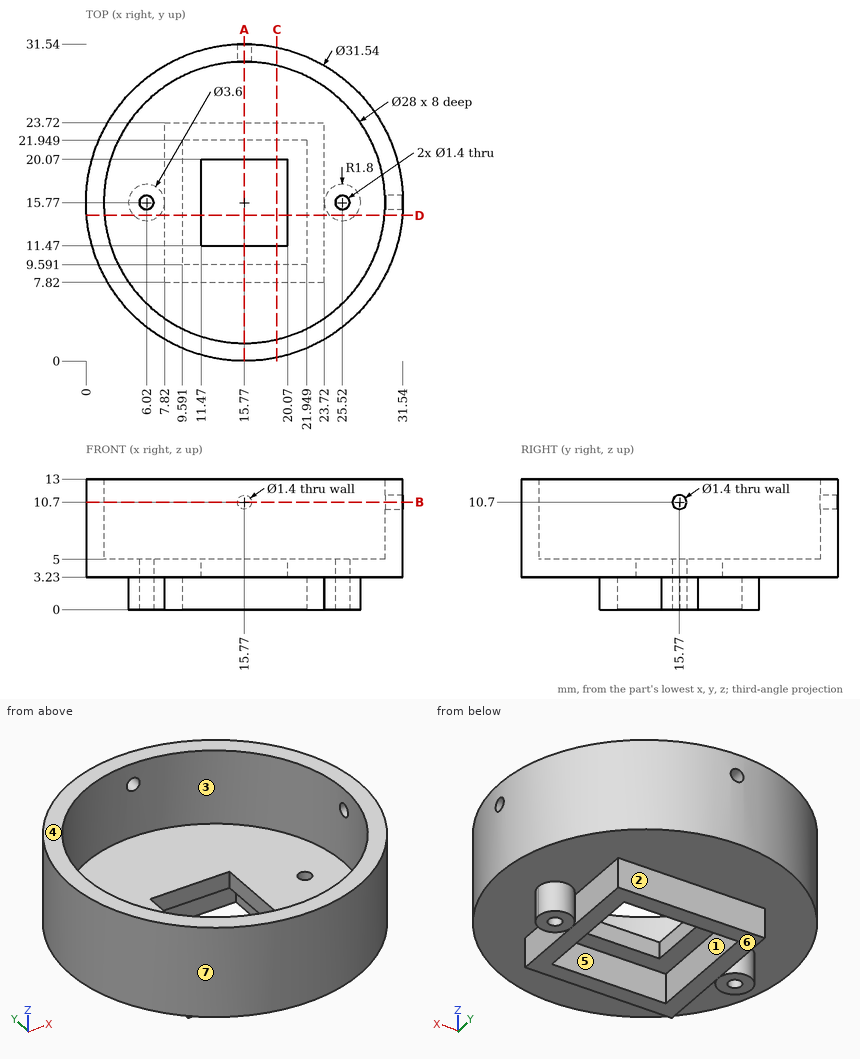
Answer from the drawing. Dimensions are ordinates in mm from the lowest x, y and z of the part. A direction names the side the tool comes from. Round coordinates to 2 decimals unless told otherwise and drop trailing zeros. Write each loop counter-clockwise with the first axis right and the second up, starting at its lowest first coordinate (ties: lowest second). Pieces come first, ordered by that corner, then holes. Notation, with made-up numbers: (3, 17.25) -> (36, 17.25) arc R21 ccw to (36, 21.25) -> close; hole circle Ø4 at (81.25, -18.5). An arc over 180 degrees is marked (long way). Answer in a Markdown table with one row per item. Add a question column.
1) Given P1, Ø4, axis at x = 26.5, y = 20.5, coming from the -Z side; P2, Ø2.5, axis at y = 13.5, z = 1.5, coming from the -X side; P3, Ø2, axis at x = 25.52, y = 15.77, coming from the +Z side; P4, Ø1.5, axis at y = 26, z = 2, coming from the -X side, each flat-ended and moving along its own axis, determine where each tip first touches the part or whether it passes through.
2) Find section A-A, the plane x = 15.77. Determine the outline of the cut face in (y, z).
3) Find section D-D, the plane y = 14.5. Determine the outline of the cut face in (x, z).
4) Find section C-C, the plane x = 19. Determine the outline of the cut face in (y, z), and give its area (3 significant figures).
5) Consider line 1 (Y direction, x = 16.5, z = 3); line 2 (Z direction, x = 15.77, y = 30.3); line 3 (Z direction, x = 21.5, y = 2). Determine where each line is inside the solid, lowest interval first.
6) Determine the mould class of the marked faces 5, 6 and 7 for opening direction X: pulls with the +X half, pulls with the -X half, needs draft (parallel to the pull), parting line crosses it, or undercut.
7) Which of the six approach directions +Z, -Z, +X, -X, +Y, -Y give full straight-line access (tool end or side, diameter ignored) to the marked faces 1, 2, 3 and 4?
8) Find section B-B, the plane z = 10.7. Determine the outline of the cut face in (x, y).
Findings below:
| question | item | result |
|---|---|---|
| 1 | P1 | z = 3.23 |
| 1 | P2 | x = 4.54 |
| 1 | P3 | z = 5 |
| 1 | P4 | through |
| 2 | outline | (0, 3.23) -> (7.82, 3.23) -> (7.82, 0) -> (9.59, 0) -> (9.59, 3.23) -> (11.47, 3.23) -> (11.47, 5) -> (1.77, 5) -> (1.77, 13) -> (0, 13) -> close; (20.07, 3.23) -> (21.95, 3.23) -> (21.95, 0) -> (23.72, 0) -> (23.72, 3.23) -> (31.54, 3.23) -> (31.54, 10) -> (29.77, 10) -> (29.77, 5) -> (20.07, 5) -> close; (29.77, 11.4) -> (31.54, 11.4) -> (31.54, 13) -> (29.77, 13) -> close |
| 3 | outline | (0.05, 3.23) -> (4.74, 3.23) -> (4.74, 0) -> (7.3, 0) -> (7.3, 3.23) -> (7.82, 3.23) -> (7.82, 0) -> (9.59, 0) -> (9.59, 3.23) -> (11.47, 3.23) -> (11.47, 5) -> (1.83, 5) -> (1.83, 13) -> (0.05, 13) -> close; (20.07, 3.23) -> (21.95, 3.23) -> (21.95, 0) -> (23.72, 0) -> (23.72, 3.23) -> (24.24, 3.23) -> (24.24, 0) -> (26.8, 0) -> (26.8, 3.23) -> (31.49, 3.23) -> (31.49, 13) -> (29.71, 13) -> (29.71, 5) -> (20.07, 5) -> close |
| 4 | outline | (0.33, 3.23) -> (7.82, 3.23) -> (7.82, 0) -> (9.59, 0) -> (9.59, 3.23) -> (11.47, 3.23) -> (11.47, 5) -> (2.15, 5) -> (2.15, 13) -> (0.33, 13) -> close; (20.07, 3.23) -> (21.95, 3.23) -> (21.95, 0) -> (23.72, 0) -> (23.72, 3.23) -> (31.21, 3.23) -> (31.21, 13) -> (29.39, 13) -> (29.39, 5) -> (20.07, 5) -> close |
| 4 | area | 79.9 mm² |
| 5 | line 1 | 7.82 to 9.59, 21.95 to 23.72 |
| 5 | line 2 | 3.23 to 10, 11.4 to 13 |
| 5 | line 3 | 3.23 to 13 |
| 6 | face 5 | undercut |
| 6 | face 6 | needs draft |
| 6 | face 7 | parting line crosses it |
| 7 | face 1 | -Z |
| 7 | face 2 | -Z, +X, -X, +Y |
| 7 | face 3 | +Z |
| 7 | face 4 | +Z, +X, -X, +Y, -Y |
| 8 | outline | (15.07, 29.75) -> (15.07, 31.52) arc R15.77 ccw (long way) to (31.52, 15.07) -> (29.75, 15.07) arc R14 cw (long way) to start; (16.47, 29.75) arc R14 cw to (29.75, 16.47) -> (31.52, 16.47) arc R15.77 ccw to (16.47, 31.52) -> close |
